Could you check a few things on this model? Use its own coordinates, in mm. Coordinates: 2 decimals unless noted, no trailing zeros. Write each loop counter-clockwise with the first axis right and the second up, starting at its lowest first coordinate (ties: lowest second). Pieces come first, ordered by that corner, then holes. Notation, with made-up numbers: (-16.5, 83.25) - (1.5, 83.25) arc R20 ccw to (1.5, 121.25) - close; hole circle Ø10 at (60, 68.25). An arc over 180 degrees is marked (long way). Answer as a JSON object with one key per item and string values. Group by question number.
1) Will these pins go through, and if not, where does the flat tip stop? pin 1 Ø1.5 at (x, z) = (-9, 1.5) entering from -Y; pin 2 Ø3 at (y, z) = (-8, 0.5) entering from -X; pin 3 Ø2 at (y, z) = (-9.5, 5.5) entering from +X.
2) If we section it at B-B (x = 0): Write out the boundary of the cut face in (y, z), plus the area to 4 significant figures.
3) If we section it at C-C (z = 1.5): Write out the boundary of the cut face in (x, y).
4) Please list where these lines run through material, in increasing order: line 1 along Y through (x, z) = (0, 1.5); line 2 along X through (y, z) = (-5.5, 0.75); line 3 along X through (y, z) = (-5.75, 4.75).
5) If we section it at D-D (y = -6): Write out the boundary of the cut face in (x, z), plus the area to 3 significant figures.
6) If we section it at A-A (y = 12): Write out the boundary of the cut face in (x, z).
7) We'd pull the mould along X, two halves only. Please class faces 1 (the flat face through (3, 0, 0)), 2 (the cylindrical face through (-14.985, 0.66, 3.451)), 3 (the cylindrical face through (0.54, -2.44, 3.45)): released by +X, released by -X, zero draft, split by the parting line, or undercut.
```python
from build123d import *

# Parameters (mm, degrees)
SKETCH1_R           = 15
BOSS_EXTRUDE2_DEPTH = 7
SKETCH2_R           = 2.5
CUT_EXTRUDE1_DEPTH  = 7
SKETCH3_R           = 1.25
CUT_EXTRUDE2_DEPTH  = 23.338307904


with BuildPart() as part:
    # Sketch1 → Boss-Extrude2 (new body)
    with BuildSketch(Plane.XY):
        Circle(SKETCH1_R)
    extrude(amount=BOSS_EXTRUDE2_DEPTH)

    # Sketch2 → Cut-Extrude1 (cut)
    with BuildSketch(Plane(origin=(0, 0, 0), x_dir=(-1, 0, 0), z_dir=(0, 0, -1))):
        Circle(SKETCH2_R)
    extrude(amount=-CUT_EXTRUDE1_DEPTH, mode=Mode.SUBTRACT)

    # Sketch3 → Cut-Extrude2 (cut, through all)
    with BuildSketch(Plane.XY.offset(7)):
        with Locations((0, 12)):
            Circle(SKETCH3_R)
        with Locations((10.392304845, -6)):
            Circle(SKETCH3_R)
        with Locations((-10.392304845, -6)):
            Circle(SKETCH3_R)
    extrude(amount=-CUT_EXTRUDE2_DEPTH, mode=Mode.SUBTRACT)


solid = part.part
```
Here are the results:
{
 "1": {"pin 1": "stops at y = -12.53", "pin 2": "stops at x = -13.52", "pin 3": "stops at x = 12.36"},
 "2": {"outline": "(-15, 0) - (-2.5, 0) - (-2.5, 7) - (-15, 7) - close; (2.5, 0) - (10.75, 0) - (10.75, 7) - (2.5, 7) - close; (13.25, 0) - (15, 0) - (15, 7) - (13.25, 7) - close", "area": "157.5 mm²"},
 "3": {"outline": "circle Ø30 at (0, 0); hole circle Ø2.5 at (-10.39, -6); hole circle Ø5 at (0, 0); hole circle Ø2.5 at (0, 12); hole circle Ø2.5 at (10.39, -6)"},
 "4": {"line 1": "y = -15 to -2.5, 2.5 to 10.75, 13.25 to 15", "line 2": "x = -13.96 to -11.54, -9.25 to 9.25, 11.54 to 13.96", "line 3": "x = -13.85 to -11.62, -9.17 to 9.17, 11.62 to 13.85"},
 "5": {"outline": "(-13.75, 0) - (-11.64, 0) - (-11.64, 7) - (-13.75, 7) - close; (-9.14, 0) - (9.14, 0) - (9.14, 7) - (-9.14, 7) - close; (11.64, 0) - (13.75, 0) - (13.75, 7) - (11.64, 7) - close", "area": "157 mm²"},
 "6": {"outline": "(-9, 0) - (-1.25, 0) - (-1.25, 7) - (-9, 7) - close; (1.25, 0) - (9, 0) - (9, 7) - (1.25, 7) - close"},
 "7": {"face 1": "zero draft", "face 2": "split by the parting line", "face 3": "undercut"}
}
